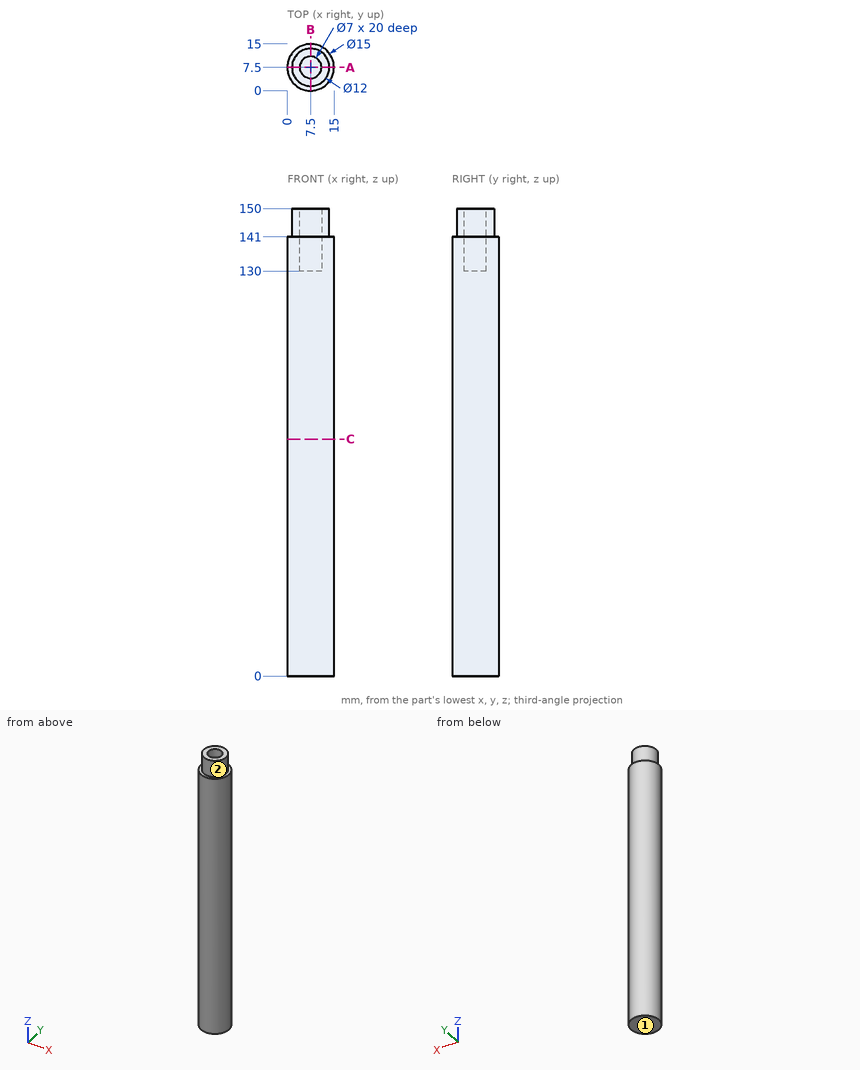
Could you check a few things on this drawing? It's one solid part, dimensions in mm from its lowest x, y, z. A direction names the side the tool comes from. Round coordinates to 2 decimals unless told otherwise and drop trailing zeros. Order: outer loops, then holes, each group sorted by start corner. A loop starts at its lowest first (then second) coordinate and runs counter-clockwise, first axis right, second up. Notation, with made-up numbers: M 75,85.5 L 99,85.5 A30 ccw 99,108.5 Z; hole C -27.5,80 d6. An arc over 180 degrees is marked long. One line per question, with ' | ' between items. Start each with the question number.
(1) Please list where these lines run through material, in increasing order: line 1 along Y through (x, z) = (7.5, 143); line 2 along Z through (x, y) = (4.5, 6.25); line 3 along Y through (x, z) = (12, 66).
(2) Suppose I cut it at A-A on y = 7.5. List the corners of the cut face in (x, z) for me.
(3) For the marked faces 1 and 2, which set-ups out of +Z, -Z, +X, -X, +Y, -Y let a thin tool reach every point of the face, with its end or its side?
(4) For P1, Ø4, axis at x = 7.5, y = 7.5, coming from the +Z side; P2, Ø1, axis at y = 4, z = 67.5, coming from the +X side; P3, Ø4, axis at y = 12.5, z = 132.5, coming from the -X side, each with a flat end and sliding along its axis, tell me the tip position at first contact or that it passes through.
(5) Suppose I cut it at C-C on z = 76. List the corners of the cut face in (x, y) for me, then the cut area to 3 significant figures.
Geometry results:
1) line 1: 1.5 to 4, 11 to 13.5 | line 2: 0 to 130 | line 3: 1.5 to 13.5
2) outline: M 0,0 L 15,0 L 15,141 L 13.5,141 L 13.5,150 L 11,150 L 11,130 L 4,130 L 4,150 L 1.5,150 L 1.5,141 L 0,141 Z
3) face 1: -Z, +X, -X, +Y, -Y | face 2: +Z
4) P1: z = 130 | P2: x = 14.37 | P3: x = 0.63
5) outline: C 7.5,7.5 d15 | area: 177 mm²
